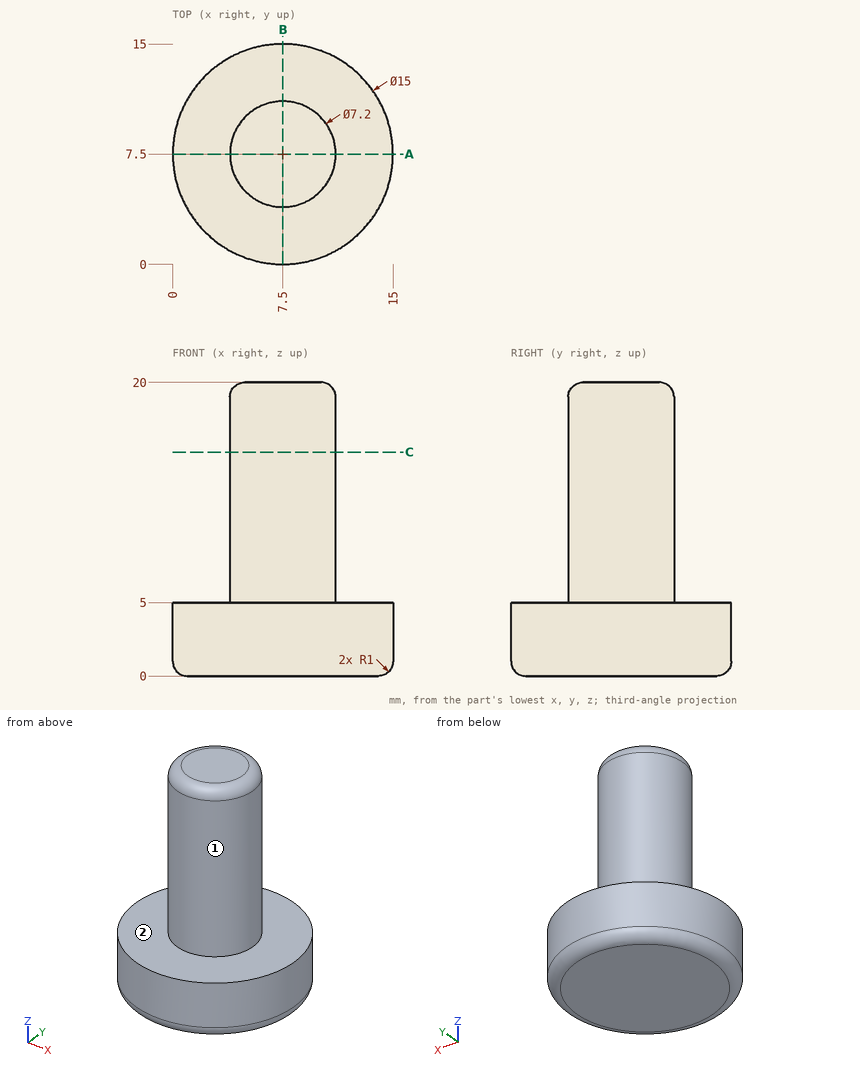
Study the drawing (mm; zero at the part's minimum x, y, z) and answer. Give positions to 0.01 mm unless a question says otherwise; leave off trailing zeros. Loops run counter-clockwise (first coordinate to the right, second up) from the corner with the lowest first, then second, coordinate; pieces in that order, holes last. Notation, with made-up numbers: (9, 57.5) - (17, 57.5) arc R26 cw to (17, 91.5) - close; hole circle Ø4 at (14, 30). An arc over 180 degrees is marked (long way). Answer as CSV lines item,"result". Start each with the question number.
1) Determine the mould class of the marked faces 1 and 2 for opening direction Y: released by +Y, released by -Y, zero draft, split by the parting line, or undercut.
2) Each of these flat-tipped pins is pushed along its axis until it touches: pin 1 Ø2 at (x, y) = (6, 3) entering from -Z; pin 2 Ø5 at (x, z) = (8.5, 12.5) entering from -Y; pin 3 Ø5 at (x, z) = (3.5, 6.5) entering from +Y; pin 4 Ø6 at (x, y) = (13.5, 8) entering from +Z. Where does it stop, or does it pass through?
3) Find section C-C (z = 15.25). Write down the section's boundary in (x, y).
4) Straight lines are drawn through the part: L1, parallel to Z at x = 10, y = 10.25; L2, parallel to Y at x = 5.25, z = 10.75; L3, parallel to Y at x = 10.5, z = 5.75. For each, find the intervals that lie inside material, in ascending order. Write a range as from..to.
5) Find section A-A (y = 7.5). Write down the section's boundary in (x, z).
Findings below:
1,face 1,"split by the parting line"
1,face 2,"zero draft"
2,pin 1,"z = 0"
2,pin 2,"y = 3.9"
2,pin 3,"y = 14.73"
2,pin 4,"z = 19.91"
3,outline,"circle Ø7.2 at (7.5, 7.5)"
4,L1,"0..5"
4,L2,"4.69..10.31"
4,L3,"5.51..9.49"
5,outline,"(0, 1) arc R1 ccw to (1, 0) - (14, 0) arc R1 ccw to (15, 1) - (15, 5) - (11.1, 5) - (11.1, 19) arc R1 ccw to (10.1, 20) - (4.9, 20) arc R1 ccw to (3.9, 19) - (3.9, 5) - (0, 5) - close"
